Work out the finished part from the listing and answer in its coordinate system (mm). Face numbers are marked on the shaded views. A direction names the side the tool comes from. Coordinates: 2 decimals unless noted, no trailing zeros. Loops run counter-clockwise (first coordinate to the right, second up) from the corner with the lowest first, then second, coordinate; pieces in that order, holes last. Notation, with made-up numbers: (23.25, 73.25) -> (75.25, 73.25) arc R34 cw to (75.25, 109.25) -> close; hole circle Ø8 at (32, 30.5). An arc over 180 degrees is marked (long way). Use a Markdown table: item, result.
from build123d import *

# Parameters (mm, degrees)
F0_W            = 160
F0_H            = 86
F1_DEPTH        = 15
F3_DEPTH        = 18
F4_R            = 8
F6_D            = 11
F9_DEPTH        = 14
F11_D           = 8
F12_C1_SIZE2    = 13
F12_C1_SIZE     = 40
F12_C2_SIZE2    = 40
F12_C2_SIZE     = 13
F16_D           = 6
F16_DEPTH       = 12
F16_START       = 0.2837665
F16_TIP         = 1.8025818571
F18_D           = 11
F20_D           = 11
F20_CBORE_D     = 16
F20_CBORE_DEPTH = 4


# Not quite as in the source:
# - two fillets or chamfers of one size are made in one step
# - a pattern or mirror of a feature is missing from the dataset's text; its kind, count and spacing are read off the source's solid


with BuildPart() as f1:
    # F0 (on Top) → F1 (new body)
    with BuildSketch(Plane.XY):
        Rectangle(F0_W, F0_H)
    extrude(amount=F1_DEPTH)

    # F2 (on face) → F3 (join)
    with BuildSketch(Plane.XZ.offset(43)):
        with BuildLine():
            Line((48, 45), (-34.4243225836, 15))
            Line((-34.4243225836, 15), (80, 15))
            Line((80, 15), (80, 53))
            ThreePointArc((80, 53), (64, 69), (48, 53))
            Line((48, 53), (48, 45))
        make_face()
    f3 = extrude(amount=-F3_DEPTH)

    # F3_copies: F3 across plane
    add(f3.mirror(Plane.ZX))

    # F4
    f4_edges = [f1.edges().sort_by_distance(p)[0] for p in [
        (48, -34, 45),
        (48, 34, 45),
    ]]
    fillet(f4_edges, radius=F4_R)

    # F6 (through all)
    with Locations(Plane.XZ.offset(43)):
        with Locations((64, 53)):
            Hole(F6_D / 2)

    # F8 (on offset) → F9 (join)
    with BuildSketch(Plane.XZ.offset(30)):
        with BuildLine():
            Line((-80, 25), (-80, 15))
            Line((-80, 15), (-61, 15))
            Line((-61, 15), (-61, 25))
            ThreePointArc((-61, 25), (-70.5, 34.5), (-80, 25))
        make_face()
    f9 = extrude(amount=-F9_DEPTH)

    # F9_copies: F9 across plane
    add(f9.mirror(Plane.ZX))

    # F11 (through all)
    with Locations(Plane.XZ.offset(30)):
        with Locations((-70.5, 25)):
            Hole(F11_D / 2)

    # F12: chamfer of 40 x 13 on 2 edges, made by hand

    # F12_c1
    f12_c1_edges = [f1.edges().sort_by_distance(p)[0] for p in [
        (-80, -43, 7.5),
    ]]
    f12_c1_side = f1.faces().sort_by_distance((-79.74, -43, 7.5))[0]
    chamfer(f12_c1_edges, length=F12_C1_SIZE, length2=F12_C1_SIZE2, reference=f12_c1_side)

    # F12_c2
    f12_c2_edges = [f1.edges().sort_by_distance(p)[0] for p in [
        (-80, 43, 7.5),
    ]]
    f12_c2_side = f1.faces().sort_by_distance((-80, 42.74, 7.5))[0]
    chamfer(f12_c2_edges, length=F12_C2_SIZE, length2=F12_C2_SIZE2, reference=f12_c2_side)

    # F16
    # its depths count from where the whole tool has entered the part; down to there all is cleared
    with Locations(Plane.XY.offset(69).offset(-F16_START)):
        with Locations((64, -34), (64, 34)):
            Hole(F16_D / 2, depth=F16_DEPTH)
            with Locations((0, 0, -(F16_DEPTH + F16_TIP / 2))):  # 118° drill point
                Cone(0, F16_D / 2, F16_TIP, mode=Mode.SUBTRACT)

    # F18 (through all)
    with Locations(Plane.XY.offset(15)):
        with Locations((-47, -16), (-47, 16)):
            Hole(F18_D / 2)

    # F20 (through all)
    with Locations(Plane.XY.offset(15)):
        with Locations((64, 0)):
            CounterBoreHole(F20_D / 2, F20_CBORE_D / 2, F20_CBORE_DEPTH)


solid = f1.part
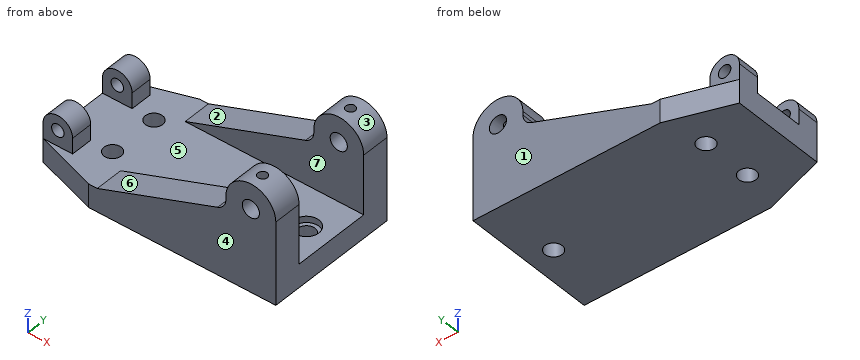
Q1. Section B-B on y = 0 is taken. Determine the outline of the cut face in (x, z), and give its area (4 significant figures).
Solved:
| item | result |
|---|---|
| outline | (-80, 0) -> (58.5, 0) -> (58.5, 11) -> (56, 11) -> (56, 15) -> (-80, 15) -> close; (69.5, 0) -> (80, 0) -> (80, 15) -> (72, 15) -> (72, 11) -> (69.5, 11) -> close |
| area | 2,215 mm² |
Q2. Section C-C on x = -47 is taken. Determine the outline of the cut face in (y, z) (3 decimals).
Solved:
| item | result |
|---|---|
| outline | (-40.725, 0) -> (-21.5, 0) -> (-21.5, 15) -> (-40.725, 15) -> close; (-10.5, 0) -> (10.5, 0) -> (10.5, 15) -> (-10.5, 15) -> close; (21.5, 0) -> (40.725, 0) -> (40.725, 15) -> (21.5, 15) -> close |
Q3. Determine the mould class of the marked faces 1, 2 and 3 for opening direction X: pulls with the +X half, pulls with the -X half, needs draft (parallel to the pull), parting line crosses it, or undercut.
Solved:
| item | result |
|---|---|
| face 1 | needs draft |
| face 2 | undercut |
| face 3 | parting line crosses it |
Q4. Given pin 1 Ø1.9 at (y, z) = (35.5, 51.5) entering from -X; pin 2 Ø3 at (y, z) = (20, 21.5) entering from +X; pin 3 Ø2 at (x, y) = (-28.5, 25.5) entering from +Z; pin 4 Ø7 at (x, z) = (-70.5, 25) entering from -Y, each flat-ended and moving along its own axis, determine where each tip first touches the part or whether it passes through.
Solved:
| item | result |
|---|---|
| pin 1 | x = 48 |
| pin 2 | x = -61 |
| pin 3 | z = 17.52 |
| pin 4 | through |
Q5. For the marked faces 4, 5, 6 and 7, determine the directions among +Z, -Z, +X, -X, +Y, -Y from which every point of the face is accessible in a straight line to the end or side of a thin tool.
Solved:
| item | result |
|---|---|
| face 4 | +Z, -Z, +X, -X, -Y |
| face 5 | +Z |
| face 6 | +Z, +Y, -Y |
| face 7 | +Z, +X |
Q6. Section A-A on z = 64 is taken. Determine the outline of the cut face in (x, y).
Solved:
| item | result |
|---|---|
| outline | (52.38, -43) -> (75.62, -43) -> (75.62, -25) -> (52.38, -25) -> close; (52.38, 25) -> (75.62, 25) -> (75.62, 43) -> (52.38, 43) -> close; hole circle Ø6 at (64, -34); hole circle Ø6 at (64, 34) |
Q7. Section D-D on x = -22 is taken. Determine the outline of the cut face in (y, z), and give its area (3 significant figures).
Solved:
| item | result |
|---|---|
| outline | (-43, 0) -> (43, 0) -> (43, 19.52) -> (25, 19.52) -> (25, 15) -> (-25, 15) -> (-25, 19.52) -> (-43, 19.52) -> close |
| area | 1,450 mm² |
Q8. Consider line 1 (Y direction, x = 51.5, z = 18); line 2 (Z direction, x = -70.5, y = -26.5); line 3 (Z direction, x = 64, y = -37.25). Determine where each line is inside the solid, lowest interval first. Write a range as [from, to].
Solved:
| item | result |
|---|---|
| line 1 | [-43, -25], [25, 43] |
| line 2 | [0, 21], [29, 34.5] |
| line 3 | [0, 47.5], [58.5, 69] |
